Read the model definition and answer for the solid it produces. Units are mm, in the model's axes. A direction names the side the tool comes from. Round coordinates to 2 decimals unless told otherwise and drop trailing zeros. Order: outer loops, then holes, each group sorted by start corner. A loop starts at its lowest first (then second) coordinate and runs counter-clockwise, first axis right, second up. Notation, with made-up numbers: (-35.75, 54) -> (23.25, 54) arc R23 cw to (23.25, 67) -> close; hole circle Ø1 at (-31.5, -33). An arc over 180 degrees is marked (long way). Answer as a JSON object with one key per item and string values. Group by question number.
Item 1: Section D-D, the plane x = 5 is taken. Write down the section's boundary in (y, z) (3 decimals), plus the area to 3 significant figures.
Item 2: Section C-C, the plane z = 15.24 is taken. Write down the section's boundary in (x, y) (1 decimal).
Item 3: Consider probe 1 along X at (y, z) = (2, 6); probe 2 along Y at (x, z) = (-0.1, 15.24) (3 decimals); probe 3 along X at (y, z) = (1, 6). Determine where each line is inside the solid, lowest interval first. Write a range as from..to.
Item 4: For faces 1 (the cylindrical face through (-0.022, -42.183, 11.683)), 2 (the flat face through (16, 0, 15)), 3 (the flat face through (-1.588, -21, 15)), determine the directions among +Z, -Z, +X, -X, +Y, -Y from which every point of the face is accessible in a straight line to the end or side of a thin tool.
Item 5: Section A-A, the plane z = 24.13 is taken. Write down the section's boundary in (x, y) (1 decimal).
Item 6: Section B-B, the plane z = 2 is taken. Write down the section's boundary in (x, y) (1 decimal).
Item 7: The mould has two halves that part along Z. Classify faces 4 (the flat face through (0, -42.545, 25)), 5 (the cylindrical face through (-0.022, -42.163, 18.777)), 6 (the flat face through (1, -11, 30.48)): pulls with the +Z half, pulls with the -Z half, needs draft (parallel to the pull), parting line crosses it, or undercut.
Item 8: Given P1, Ø10, axis at x = 16.5, z = 18, coming from the -Y side; P2, Ø8, axis at y = -37, z = 24.5, coming from the +X side, each flat-ended and moving along its own axis, determine where each tip first touches the part or whether it passes through.
from build123d import *

# Parameters (mm, degrees)
BOSS_EXTRUDE1_DEPTH          = 30.48
FILLET1_R                    = 2.54
F_3_0_3_DIAMETER_HOLE2_D     = 3
F_3_0_3_DIAMETER_HOLE2_DEPTH = 3.175
F_3_0_3_DIAMETER_HOLE1_D     = 3
F_3_0_3_DIAMETER_HOLE1_DEPTH = 3.175
CUT_EXTRUDE1_DEPTH           = 3.175
FILLET2_R                    = 1.27


with BuildPart() as part:
    # Sketch1 → Boss-Extrude1 (new body)
    with BuildSketch(Plane.XY):
        Polygon((-1.5875, 3.175), (-1.5875, -42.545), (1.5875, -42.545), (1.5875, 0), (28.8925, 0), (28.8925, 3.175), align=None)
    extrude(amount=BOSS_EXTRUDE1_DEPTH)

    # Fillet1
    fillet1_edges = [part.edges().sort_by_distance(p)[0] for p in [
        (1.5875, 0, 15.24),
        (-1.5875, 3.175, 15.24),
    ]]
    fillet(fillet1_edges, radius=FILLET1_R)

    # Ø3.0 (3) Diameter Hole2
    with Locations(Plane(origin=(1.5875, 0, 0), x_dir=(0, 0, -1), z_dir=(1, 0, 0))):
        with Locations((-15.24, -15.6591), (-15.24, -25.4381)):
            Hole(F_3_0_3_DIAMETER_HOLE2_D / 2, depth=F_3_0_3_DIAMETER_HOLE2_DEPTH)

    # Ø3.0 (3) Diameter Hole1
    with Locations(Plane(origin=(0, 0, 0), x_dir=(-1, 0, 0), z_dir=(0, -1, 0))):
        with Locations((-22.5425, -6.35), (-9.8425, -6.35), (-9.8425, -24.13), (-22.5425, -24.13)):
            Hole(F_3_0_3_DIAMETER_HOLE1_D / 2, depth=F_3_0_3_DIAMETER_HOLE1_DEPTH)

    # Sketch7 → Cut-Extrude1 (cut)
    with BuildSketch(Plane(origin=(1.5875, 0, 0), x_dir=(0, 0, -1), z_dir=(1, 0, 0))):
        with BuildLine():
            Line((-18.415, -42.545), (-18.415, -35.317518126))
            ThreePointArc((-18.415, -35.317518126), (-15.24, -32.385), (-12.065, -35.317518126))
            Line((-12.065, -35.317518126), (-12.065, -42.545))
            Line((-12.065, -42.545), (-18.415, -42.545))
        make_face()
    extrude(amount=-CUT_EXTRUDE1_DEPTH, mode=Mode.SUBTRACT)

    # Fillet2
    fillet2_edges = [part.edges().sort_by_distance(p)[0] for p in [
        (0, -42.545, 12.065),
        (0, -42.545, 18.415),
    ]]
    fillet(fillet2_edges, radius=FILLET2_R)


solid = part.part
Values found:
{
 "1": {"outline": "(0, 0) -> (3.175, 0) -> (3.175, 30.48) -> (0, 30.48) -> close", "area": "96.8 mm2"},
 "2": {"outline": "(-1.6, -32.4) -> (1.6, -32.4) -> (1.6, -26.9) -> (-1.6, -26.9) -> close; (-1.6, -23.9) -> (1.6, -23.9) -> (1.6, -17.2) -> (-1.6, -17.2) -> close; (-1.6, -14.2) -> (1.6, -14.2) -> (1.6, -2.5) arc R2.5 cw to (4.1, 0) -> (28.9, 0) -> (28.9, 3.2) -> (1, 3.2) arc R2.5 ccw to (-1.6, 0.6) -> close"},
 "3": {"probe 1": "-1.19..8.38, 11.3..21.08, 24..28.89", "probe 2": "-32.385..-26.938, -23.938..-17.159, -14.159..2.947", "probe 3": "-1.56..8.38, 11.3..21.08, 24..28.89"},
 "4": {"face 1": "+X, -X, -Y", "face 2": "+Z, -Z, +X, -Y", "face 3": "+Z, -Z, -X, +Y, -Y"},
 "5": {"outline": "(-1.6, -42.5) -> (1.6, -42.5) -> (1.6, -2.5) arc R2.5 cw to (4.1, 0) -> (8.3, 0) -> (8.3, 3.2) -> (1, 3.2) arc R2.5 ccw to (-1.6, 0.6) -> close; (11.3, 0) -> (21, 0) -> (21, 3.2) -> (11.3, 3.2) -> close; (24, 0) -> (28.9, 0) -> (28.9, 3.2) -> (24, 3.2) -> close"},
 "6": {"outline": "(-1.6, -42.5) -> (1.6, -42.5) -> (1.6, -2.5) arc R2.5 cw to (4.1, 0) -> (28.9, 0) -> (28.9, 3.2) -> (1, 3.2) arc R2.5 ccw to (-1.6, 0.6) -> close"},
 "7": {"face 4": "needs draft", "face 5": "undercut", "face 6": "pulls with the +Z half"},
 "8": {"P1": "y = 0", "P2": "x = 1.59"}
}
